Build history of the part. All positions in model axes, mm. A direction names the side the tool comes from. Round coordinates to 2 decimals unless told otherwise and drop trailing zeros. Order: outer loops, then holes, each group sorted by start corner. A loop starts at its lowest first (then second) coordinate and runs counter-clockwise, first axis right, second up. Notation, with made-up numbers: M 54.5,23.5 L 98.5,23.5 A23 cw 98.5,34.5 Z; hole C -35.5,48.25 d2. An arc over 180 degrees is marked long. One line per item, written item: value. Start each with the question number.
Item 1: Band-saw the part on C-C, the plane y = 2.5. Write the cut outline in (x, z), then the cut area to 3 significant figures.
Item 2: Pin check, flat tips, straight feed: pin 1 (5 mm diameter, centred on x = -4, y = 8.5, fed in from +Z); pin 2 (2.5 mm diameter, centred on x = 0, z = -1.5, fed in from +Y); pin 3 (0.7 mm diameter, centred on x = 5, y = -1, fed in from +Z) (3 decimals). Stop position of each tip, or through.
Item 3: Tool access for faces 1 (the flat face through (4.625, -1, 5)), 2 (the flat face through (0, 7.8, 0)), 3 (the flat face through (-5.475, -1, -5)), 4 (the cylindrical face through (-0.108, -1.085, -0.488)): list every direction of +Z, -Z, +X, -X, +Y, -Y with a clear straight run to the whole face (end or side of a thin tool).
Item 4: Probe L1, parallel to Z at x = 0, y = 8.9; L2, parallel to X at y = 9.9, z = 0; L3, parallel to X at y = 8.75, z = -0.75. List the from-to ranges inside material, lowest first.
Item 5: Band-saw the part on A-A, the plane y = 6. Write the cut outline in (x, z), then the cut area to 3 significant figures.
Item 6: Two-plate mould, pull along Y, no slides. Class faces 5 (the cylindrical face through (-0.03, 6.3, 4.68)), 6 (the flat face through (5.475, -1, 5)), 7 (the flat face through (-2, 5, 2)), 8 (the flat face through (0, 10, 4.5)): +Y half, -Y half, draft (parallel to the pull), parting line (faces both ways), or undercut.
```python
from build123d import *

# Parameters (mm, degrees)
ESQUISSE2_W                  = 22
ESQUISSE2_H                  = 22
ESQUISSE2_W_2                = 12
ESQUISSE2_H_2                = 12
ENL_V_MAT_EXTRU_4_DEPTH      = 14
ENL_V_MAT_EXTRU_4_DEPTH_BACK = 1
ESQUISSE3_W                  = 0.85
ESQUISSE3_H                  = 0.85
BOSS_EXTRU_1_DEPTH           = 2.2
ESQUISSE4_R                  = 0.6
ENL_V_MAT_EXTRU_5_DEPTH      = 2
ESQUISSE5_R                  = 2.2
ENL_V_MAT_EXTRU_6_DEPTH      = 1.5
ESQUISSE6_R                  = 1
BOSS_EXTRU_2_DEPTH           = 1
ESQUISSE7_R                  = 0.5
BOSS_EXTRU_3_DEPTH           = 2.4
CHANFREIN1_SIZE              = 0.2


with BuildPart() as part:
    # Esquisse1 → Révolution1 (revolve)
    with BuildSketch(Plane.XY):
        with BuildLine():
            Line((0, 0), (-10, 0))
            Line((-10, 0), (-10, 0.820061659))
            Line((-10, 0.820061659), (-4.85, 2.2))
            Line((-4.85, 2.2), (-4.85, 7.701564029))
            ThreePointArc((-4.85, 7.701564029), (-4.6, 8.5), (-4.85, 9.298435971))
            Line((-4.85, 9.298435971), (-4.85, 13))
            Line((-4.85, 13), (-4.15, 13))
            Line((-4.15, 13), (-4.15, 5))
            Line((-4.15, 5), (-2.5, 5))
            Line((-2.5, 5), (-2.5, 10))
            Line((-2.5, 10), (-1, 10))
            Line((-1, 10), (-1, 9.8))
            Line((-1, 9.8), (0, 9.8))
            Line((0, 9.8), (0, 0))
        make_face()
    revolve(axis=Axis((0, 9.8, 0), (0, -1, 0)))

    # Esquisse2 → Enlèv. mat.-Extru.4 (cut, two sides)
    with BuildSketch(Plane(origin=(0, 0, 0), x_dir=(1, 0, 0), z_dir=(0, 1, 0))) as enl_v_mat_extru_4_sk:
        Rectangle(ESQUISSE2_W, ESQUISSE2_H)
        Rectangle(ESQUISSE2_W_2, ESQUISSE2_H_2, mode=Mode.SUBTRACT)
    extrude(amount=ENL_V_MAT_EXTRU_4_DEPTH, mode=Mode.SUBTRACT)
    extrude(enl_v_mat_extru_4_sk.sketch, amount=-ENL_V_MAT_EXTRU_4_DEPTH_BACK, mode=Mode.SUBTRACT)

    # Esquisse3 → Boss.-Extru.1 (add)
    with BuildSketch(Plane.XZ):
        with Locations((5.05, -5.05)):
            Rectangle(ESQUISSE3_W, ESQUISSE3_H)
        with Locations((-5.05, -5.05)):
            Rectangle(ESQUISSE3_W, ESQUISSE3_H)
        with Locations((-5.05, 5.05)):
            Rectangle(ESQUISSE3_W, ESQUISSE3_H)
        with Locations((5.05, 5.05)):
            Rectangle(ESQUISSE3_W, ESQUISSE3_H)
    extrude(amount=BOSS_EXTRU_1_DEPTH)

    # Esquisse4 → Enlèv. mat.-Extru.5 (cut)
    with BuildSketch(Plane(origin=(0, 9.8, 0), x_dir=(1, 0, 0), z_dir=(0, 1, 0))):
        Circle(ESQUISSE4_R)
    extrude(amount=-ENL_V_MAT_EXTRU_5_DEPTH, mode=Mode.SUBTRACT)

    # Esquisse5 → Enlèv. mat.-Extru.6 (cut)
    with BuildSketch(Plane.XY.offset(6)):
        with Locations((0, 8.5)):
            Circle(ESQUISSE5_R)
    enl_v_mat_extru_6 = extrude(amount=-ENL_V_MAT_EXTRU_6_DEPTH, mode=Mode.SUBTRACT)

    # Esquisse6 → Boss.-Extru.2 (add)
    with BuildSketch(Plane.XY.offset(4.5)):
        with Locations((0, 8.574177758)):
            Circle(ESQUISSE6_R)
    boss_extru_2 = extrude(amount=BOSS_EXTRU_2_DEPTH)

    # Symétrie1: Enlèv. mat.-Extru.6, Boss.-Extru.2 across plane
    add(enl_v_mat_extru_6.mirror(Plane.XY), mode=Mode.SUBTRACT)
    add(boss_extru_2.mirror(Plane.XY))

    # Esquisse7 → Boss.-Extru.3 (add)
    with BuildSketch(Plane.XZ):
        Circle(ESQUISSE7_R)
    extrude(amount=BOSS_EXTRU_3_DEPTH)

    # Chanfrein1
    chanfrein1_edges = [part.edges().sort_by_distance(p)[0] for p in [
        (-0.5, -2.4, 0),
    ]]
    chamfer(chanfrein1_edges, length=CHANFREIN1_SIZE)


solid = part.part
```
Output:
1. outline: C 0,0 d9.7
1. area: 73.9 mm²
2. pin 1: stops at z = 4.5
2. pin 2: stops at y = 10
2. pin 3: stops at z = 5.475
3. face 1: +Z, -Z, -Y
3. face 2: +Y
3. face 3: +Z, -Z, -X, -Y
3. face 4: -Y
4. L1: z = -5.5 to -4.15, -2.5 to -0.6, 0.6 to 2.5, 4.15 to 5.5
4. L2: x = -4.85 to -4.15, -2.5 to -1, 1 to 2.5, 4.15 to 4.85
4. L3: x = -4.56 to -4.08, -2.38 to 2.38, 4.08 to 4.56
5. outline: C 0,0 d9.7; C 0,0 d5; hole C 0,0 d8.3
5. area: 39.4 mm²
6. face 5: undercut
6. face 6: draft
6. face 7: +Y half
6. face 8: undercut
